from build123d import *

# Parameters (mm, degrees)
BOSS_EXTRUDE1_DEPTH     = 19.05
SKETCH2_W               = 197.138384739
SKETCH2_H               = 233.965884384
CUT_EXTRUDE1_DEPTH      = 580.97531403
CUT_EXTRUDE1_DEPTH_BACK = 580.97531403


with BuildPart() as part:
    # Sketch1 → Boss-Extrude1 (new body)
    with BuildSketch(Plane.XY):
        with BuildLine():
            Line((508, 0), (-508, 0))
            ThreePointArc((-508, 0), (-520.8192309, -3.472224939), (-530.133638711, -12.93958117))
            Line((-530.133638711, -12.93958117), (-579.97531403, -101.474136014))
            Line((-579.97531403, -101.474136014), (-478.37531403, -101.474136014))
            Line((-478.37531403, -101.474136014), (-457.132157229, -63.73958117))
            ThreePointArc((-457.132157229, -63.73958117), (-447.817749418, -54.272224939), (-434.998518519, -50.8))
            Line((-434.998518519, -50.8), (434.998518519, -50.8))
            ThreePointArc((434.998518519, -50.8), (447.817749418, -54.272224939), (457.132157229, -63.73958117))
            Line((457.132157229, -63.73958117), (478.37531403, -101.474136014))
            Line((478.37531403, -101.474136014), (579.97531403, -101.474136014))
            Line((579.97531403, -101.474136014), (530.133638711, -12.93958117))
            ThreePointArc((530.133638711, -12.93958117), (520.8192309, -3.472224939), (508, 0))
        make_face()
    extrude(amount=BOSS_EXTRUDE1_DEPTH)

    # Sketch2 → Cut-Extrude1 (cut, two sides)
    with BuildSketch(Plane(origin=(0, 0, 0), x_dir=(0, 0, -1), z_dir=(1, 0, 0))) as cut_extrude1_sk:
        with Locations((-13.729414766, -53.345438188)):
            Rectangle(SKETCH2_W, SKETCH2_H)
        Polygon((0, -101.474136014), (-60.85250598, -70.206121999), (-23.664545619, 2.167536884), (37.187960361, -29.100477131), align=None, mode=Mode.SUBTRACT)
    extrude(amount=CUT_EXTRUDE1_DEPTH, mode=Mode.SUBTRACT)
    extrude(cut_extrude1_sk.sketch, amount=-CUT_EXTRUDE1_DEPTH_BACK, mode=Mode.SUBTRACT)


solid = part.part
Could you check a few things on this model? Use its own coordinates, in mm. A direction names the side the tool comes from. Coordinates: 2 decimals unless noted, no trailing zeros. Write each loop counter-clockwise with the first axis right and the second up, starting at its lowest first coordinate (ties: lowest second). Pieces come first, ordered by that corner, then holes. Notation, with made-up numbers: M 10,20 L 39,20 A25 cw 39,40 Z; hole C 81.5,-2 d1. An arc over 180 degrees is marked long. One line per question, with ' | ' between items.
1) Imagine slicing it at A-A, the plane z = 9.25. Write out the boundary of the cut face in (x, y), and give its area (3 significant figures).
Checks:
outline: M -577.3,-96.72 L -475.7,-96.72 L -457.13,-63.74 A25.4 cw -435,-50.8 L 435,-50.8 A25.4 cw 457.13,-63.74 L 475.7,-96.72 L 577.3,-96.72 L 530.13,-12.94 A25.4 ccw 523.45,-5.24 L -523.45,-5.24 A25.4 ccw -530.13,-12.94 Z | area: 58,500 mm²
2) If we mould it in two halves opening along X, with no side actions, what happens to faces 3 (the face through (526.324, -7.811, 11.508)), 4 (the face through (-6, -50.8, 9)), 5 (the face through (-8, -35, 19.05))? For each: released by +X, released by -X, zero draft, split by the parting line, or undercut.
Checks:
face 3: released by +X | face 4: undercut | face 5: zero draft
3) For pin 1 Ø1 at (x, z) = (141.5, 10.5) entering from +Y; pin 2 Ø6 at (x, z) = (-144, 13) entering from +Y; pin 3 Ø1.5 at (x, z) = (290, 13) entering from -Y, each with a flat end and sliding along its axis, tell me the tip position at first contact or that it passes through.
Checks:
pin 1: y = -4.34 | pin 2: y = -1.77 | pin 3: y = -50.8
4) For faces 1 (the face through (555.403, -57.827, 9.392)), 2 (the face through (-447.98, -54.37, 9.39)), which set-ups out of +Z, -Z, +X, -X, +Y, -Y let a thin tool reach every point of the face, with its end or its side?
Checks:
face 1: +Z, -Z, +X, +Y | face 2: +Z, -Z, -Y
5) Imagine slicing it at B-B, the plane y = -78. Write out the boundary of the cut face in (x, z).
Checks:
outline: M -566.76,0 L -465.16,0 L -465.16,19.05 L -566.76,19.05 Z; M 465.16,0 L 566.76,0 L 566.76,19.05 L 465.16,19.05 Z
6) I need wall thicknesses on probe 1 along X at (y, z) = (-78, 6); probe 2 along X at (y, z) = (-53, 14.75); probe 3 along Y at (x, z) = (526, 5.5). Which ranges of each line are inside material? Lowest first, please. Write a range as [from, to].
Checks:
probe 1: [-566.76, -465.16], [465.16, 566.76] | probe 2: [-552.69, -445.34], [445.34, 552.69] | probe 3: [-98.65, -7.48]
7) Imagine slicing it at D-D, the plane x = -196.5. Write out the boundary of the cut face in (y, z).
Checks:
outline: M -50.8,0 L -9.99,0 L -0.2,19.05 L -50.8,19.05 Z
8) Imagine slicing it at C-C, the plane x = -493. Write out the boundary of the cut face in (y, z), and give its area (3 significant figures).
Checks:
outline: M -101.47,0 L -9.99,0 L -0.2,19.05 L -91.69,19.05 Z | area: 1,740 mm²
